from build123d import *

# Parameters (mm, degrees)
SKETCH1_R           = 10.16
BOSS_EXTRUDE1_DEPTH = 1.762125
SKETCH2_R           = 8.255
BOSS_EXTRUDE2_DEPTH = 2.7305
FILLET1_R           = 1.27


with BuildPart() as part:
    # Sketch1 → Boss-Extrude1 (new, symmetric)
    with BuildSketch(Plane(origin=(0, 0, 0), x_dir=(0, 0, -1), z_dir=(1, 0, 0))):
        Circle(SKETCH1_R)
        Polygon((7.552318871, 0), (3.776159436, 6.5405), (-3.776159436, 6.5405), (-7.552318871, 0), (-3.776159436, -6.5405), (3.776159436, -6.5405), align=None, mode=Mode.SUBTRACT)
    extrude(amount=BOSS_EXTRUDE1_DEPTH, both=True)

    # Sketch2 → Boss-Extrude2 (add)
    with BuildSketch(Plane.ZY.offset(1.762125)):
        with Locations(Location((0, 0, 0), (0, 0, 180))):
            Circle(SKETCH2_R)
        Polygon((5.719231767, 0), (2.859615883, 4.953), (-2.859615883, 4.953), (-5.719231767, 0), (-2.859615883, -4.953), (2.859615883, -4.953), align=None, mode=Mode.SUBTRACT)
    extrude(amount=BOSS_EXTRUDE2_DEPTH)

    # Fillet1
    fillet1_edges = [part.edges().sort_by_distance(p)[0] for p in [
        (-1.762125, 0, 8.255),
    ]]
    fillet(fillet1_edges, radius=FILLET1_R)


solid = part.part
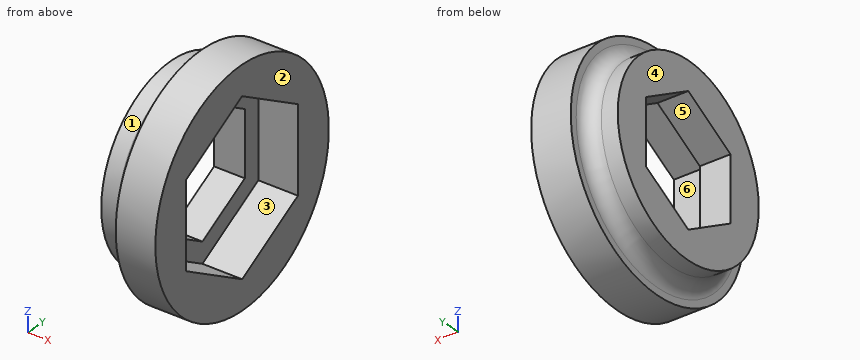
Geometry: final body of the model. Coordinates: model frame, mm. Face numbers are marked on the shaded views. A direction names the side the tool comes from. Round coordinates to 2 decimals unless told otherwise and drop trailing zeros. Loops run counter-clockwise (first coordinate to the right, second up) from the corner with the lowest first, then second, coordinate; pieces in that order, holes last. Notation, with made-up numbers: M 82,-31 L 110,-31 A25 cw 110,1 Z; hole C -13.5,-19.75 d7. An arc over 180 degrees is marked long. Put each result on its own line as item: value. Start each with the question number.
(1) Contact query for flat-ended pins moving along their axis: pin 1 Ø2 at (x, z) = (-3.5, -0.5) entering from -Y; pin 2 Ø1.5 at (x, z) = (-3, 3) entering from -Y; pin 3 Ø3 at (x, z) = (-0.5, 3.5) entering from +Y. Output: stop coordinate, or through.
(2) Set-up query: the marked faces 4, 5 and 6. Return all of +Z, -Z, +X, -X, +Y, -Y with unobstructed straight access to the full face (end or side cutting, diameter ignored); none if empty.
(3) Section query B-B (x = -1.25). Return loops of the section in (y, z).
(4) Section query A-A (z = 0). Return loops of the section in (x, y) (1 decimal), then the cut area to 3 significant figures.
(5) Draft query along Z for the marked faces 1, 2 and 3. Return one class per face: +Z half, -Z half, draft (parallel to the pull), parting line (faces both ways), or undercut.
(6) Material intervals for line 1 along Y through (x, z) = (1, 1.5); line 2 along X through (y, z) = (5.5, -1); line 3 along X through (y, z) = (-2, 9.25), sorted ascending. Write a range as [from, to].
Findings below:
1. pin 1: stops at y = -8.36
1. pin 2: stops at y = -8.04
1. pin 3: stops at y = 9.96
2. face 4: +Z, -Z, -X, +Y, -Y
2. face 5: +X, -X
2. face 6: +X
3. outline: C 0,0 d20.32; hole M -6.54,-3.78 L 0,-7.55 L 6.54,-3.78 L 6.54,3.78 L 0,7.55 L -6.54,3.78 Z
4. outline: M -4.5,-8.3 L -3,-8.3 A1.3 cw -1.8,-9.5 L -1.8,-10.2 L 1.8,-10.2 L 1.8,-6.5 L -1.8,-6.5 L -1.8,-5 L -4.5,-5 Z; M -4.5,5 L -1.8,5 L -1.8,6.5 L 1.8,6.5 L 1.8,10.2 L -1.8,10.2 L -1.8,9.5 A1.3 cw -3,8.3 L -4.5,8.3 Z
4. area: 44.2 mm2
5. face 1: parting line
5. face 2: draft
5. face 3: undercut
6. line 1: y = [-10.05, -6.54], [6.54, 10.05]
6. line 2: x = [-4.49, -1.76]
6. line 3: x = [-1.76, 1.76]
